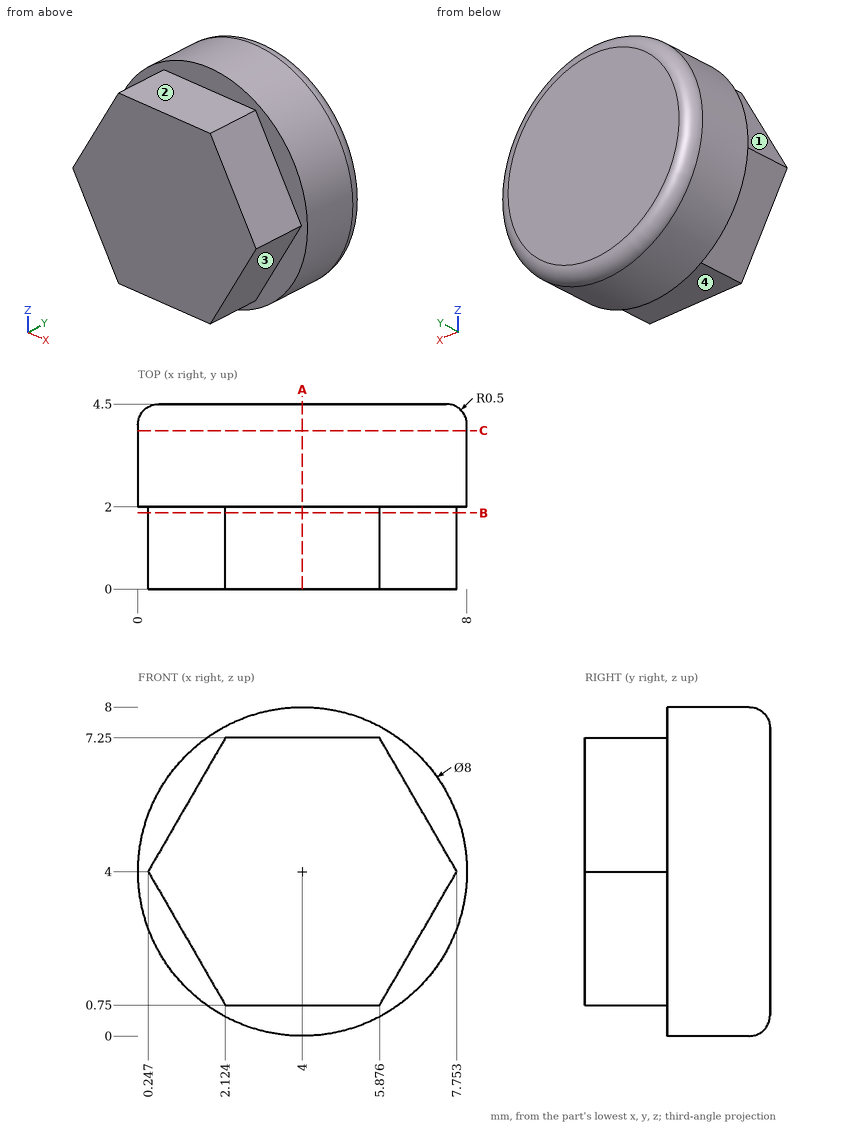
Job drawing, mm, ordinate dimensions from the low corner. One solid piece. A direction names the side the tool comes from. Coordinates: 2 decimals unless noted, no trailing zeros. Order: outer loops, then holes, each group sorted by start corner. A loop starts at its lowest first (then second) coordinate and runs counter-clockwise, first axis right, second up. Notation, with made-up numbers: M 47,86 L 52,86 A19 ccw 52,117 Z; hole C -2.75,11.5 d8. An arc over 180 degrees is marked long. One line per question, with ' | ' between items.
Q1. Slice it at B-B (y = 1.85). Give the cut face in (x, z), and give its area (3 significant figures).
A:
outline: M 0.25,4 L 2.12,0.75 L 5.88,0.75 L 7.75,4 L 5.88,7.25 L 2.12,7.25 Z | area: 36.6 mm^2
Q2. Pin check, flat tips, straight feed: P1, Ø1, axis at x = 3.5, y = 1, coming from the -Z side; P2, Ø2, axis at x = 3.5, y = 0.5, coming from the +Z side; P3, Ø1.5, axis at y = 2.5, z = 7, coming from the +X side. Stop position of each tip, or through.
A:
P1: stops at z = 0.75 | P2: stops at z = 7.25 | P3: stops at x = 7.31
Q3. 3-axis set-ups, long thin cutter, end or side, ignore diameter. For the marked faces 1, 2, 3 and 4: which of +Z, -Z, +X, -X, +Y, -Y reach the whole face in a straight line?
A:
face 1: +Z, -X, -Y | face 2: +Z, +X, -X, -Y | face 3: -Z, +X, -Y | face 4: -Z, +X, -X, -Y
Q4. Slice it at C-C (y = 3.85). Give the cut face in (x, z).
A:
outline: C 4,4 d8
Q5. Drill centre lines: line 1 (Z direction, x = 4.75, y = 1.75); line 2 (Z direction, x = 6.5, y = 4.2); line 3 (X direction, y = 2.35, z = 2.75). Where is each one in solid material? Low to high.
A:
line 1: z = 0.75 to 7.25 | line 2: z = 0.93 to 7.07 | line 3: x = 0.2 to 7.8
Q6. Slice it at A-A (x = 4). Give the cut face in (y, z), and give its area (3 significant figures).
A:
outline: M 0,0.75 L 2,0.75 L 2,0 L 4,0 A0.5 ccw 4.5,0.5 L 4.5,7.5 A0.5 ccw 4,8 L 2,8 L 2,7.25 L 0,7.25 Z | area: 32.9 mm^2
